from build123d import *
from OCP.BRepFilletAPI import BRepFilletAPI_MakeChamfer

# Parameters (mm, degrees)
SKETCH_1_W          = 60
SKETCH_1_H          = 60
EXTRUDE_1_DEPTH     = 285
CUT_EXTRUDE_1_DEPTH = 95
SKETCH_3_OUTSIDE_W  = 121.472
SKETCH_3_OUTSIDE_H  = 121.472
SKETCH_3_OUTSIDE_R  = 37.5
CUT_EXTRUDE_2_DEPTH = 289.140590684
CHAMFER_1_SIZE      = 3
CHAMFER_1_SIZE2     = 5
CHAMFER_2_SIZE      = 5


with BuildPart() as part:
    # 草图1 → 凸台-拉伸1 (new body)
    with BuildSketch(Plane.XY):
        Rectangle(SKETCH_1_W, SKETCH_1_H)
    extrude(amount=EXTRUDE_1_DEPTH)

    # 草图2 → 切除-拉伸1 (cut)
    with BuildSketch(Plane(origin=(30, 0, 0), x_dir=(0, 0, -1), z_dir=(1, 0, 0))):
        Polygon((-285, 30), (-250.358983849, -30), (-285, -30), align=None)
    extrude(amount=-CUT_EXTRUDE_1_DEPTH, mode=Mode.SUBTRACT)

    # 草图3 outside → 切除-拉伸2 (cut, through all)
    with BuildSketch(Plane(origin=(0, 0, 0), x_dir=(1, 0, 0), z_dir=(0, 0, -1))):
        Rectangle(SKETCH_3_OUTSIDE_W, SKETCH_3_OUTSIDE_H)
        Circle(SKETCH_3_OUTSIDE_R, mode=Mode.SUBTRACT)
    extrude(amount=-CUT_EXTRUDE_2_DEPTH, mode=Mode.SUBTRACT)

    # 倒角1: one chamfer whose edges measure the first distance from different faces: ONE call of the kernel's chamfer builder (chamfer() names one face for all edges)
    chamfer_1_edges_1 = [part.edges().sort_by_distance(p)[0] for p in [
        (0, -30, 250.358983849),
    ]]
    chamfer_1_side_1 = [part.faces().sort_by_distance(p)[0] for p in [
        (0, -30, 125.179491924),
    ]]
    chamfer_1_edges_2 = [part.edges().sort_by_distance(p)[0] for p in [
        (0, 30, 285),
    ]]
    chamfer_1_side_2 = [part.faces().sort_by_distance(p)[0] for p in [
        (0, 0, 267.679491924),
    ]]
    chamfer_1 = BRepFilletAPI_MakeChamfer(part.part.solid().wrapped)
    for e in chamfer_1_edges_1:
        chamfer_1.Add(CHAMFER_1_SIZE, CHAMFER_1_SIZE2, e.wrapped, chamfer_1_side_1[0].wrapped)  # the first distance lies on this face
    for e in chamfer_1_edges_2:
        chamfer_1.Add(CHAMFER_1_SIZE, CHAMFER_1_SIZE2, e.wrapped, chamfer_1_side_2[0].wrapped)  # the first distance lies on this face
    add(Compound.cast(chamfer_1.Shape()), mode=Mode.REPLACE)

    # 倒角2
    chamfer_2_edges = [part.edges().sort_by_distance(p)[0] for p in [
        (-30, 0, 0),
        (0, 30, 0),
        (30, 0, 0),
        (0, -30, 0),
        (26.516504294, -26.516504294, 0),
        (-26.516504294, 26.516504294, 0),
        (-26.516504294, -26.516504294, 0),
        (26.516504294, 26.516504294, 0),
    ]]
    chamfer(chamfer_2_edges, length=CHAMFER_2_SIZE)


solid = part.part
Read the model definition and answer for the solid it produces. Units are mm, in the model's axes. Round coordinates to 2 decimals unless told otherwise and drop trailing zeros. Loops run counter-clockwise (first coordinate to the right, second up) from the corner with the lowest first, then second, coordinate; pieces in that order, holes last. Notation, with made-up numbers: (16.5, 14) - (70.5, 14) arc R23 cw to (70.5, 37) - close; hole circle Ø11 at (15, 14). An arc over 180 degrees is marked (long way). One line per question, with ' | ' between items. Start each with the question number.
Q1. Section D-D on y = -10.5 is taken. Give the vertices of the cut face in (x, z).
Q2. Section C-C on y = 10 is taken. Give the vertices of the cut face in (x, z), plus the area to 3 significant figures.
Q3. Section A-A on x = -7.5 is taken. Give the vertices of the cut face in (y, z).
Q4. Find the intervals of material crossed by L1, parallel to X at y = -27, z = 148; L2, parallel to X at y = -24.5, z = 112; L3, parallel to Z at x = -14, y = -24, in increasing order.
Q5. A flat-ended cylindrical pin translates along its axis: pin 1 (8 mm diameter, centred on y = 23.5, z = 77.5, fed in from -X). Find the tip coordinate at first contact, or state that the pin passes through.
Q6. Section B-B on z = 29.5 is taken. Give the vertices of the cut face in (x, y).
Established:
1) outline: (-30, 5) - (-25, 0) - (25, 0) - (30, 5) - (30, 261.62) - (-30, 261.62) - close
2) outline: (-30, 5) - (-25, 0) - (25, 0) - (30, 5) - (30, 273.45) - (-30, 273.45) - close | area: 16,400 mm²
3) outline: (-30, 5) - (-25, 0) - (25, 0) - (30, 5) - (30, 280) - (27.4, 283.5) - (-25.67, 252.86) - (-30, 247.36) - close
4) L1: -26.02 to 26.02 | L2: -28.39 to 28.39 | L3: 0 to 253.82
5) pin 1: x = -30
6) outline: (-30, -22.5) arc R37.5 ccw to (-22.5, -30) - (22.5, -30) arc R37.5 ccw to (30, -22.5) - (30, 22.5) arc R37.5 ccw to (22.5, 30) - (-22.5, 30) arc R37.5 ccw to (-30, 22.5) - close
